Geometry: final body of the model. Coordinates: model frame, mm. Face numbers are marked on the shaded views. A direction names the side the tool comes from. Coordinates: 2 decimals unless noted, no trailing zeros. Write each loop counter-clockwise with the first axis right and the second up, starting at its lowest first coordinate (ties: lowest second). Pieces come first, ordered by that corner, then holes.
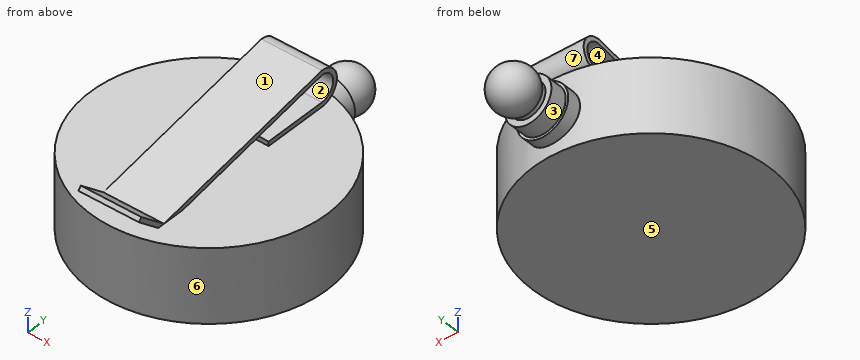
from build123d import *

# Parameters (mm, degrees)
F0_R     = 16
F1_DEPTH = 10
F3_DEPTH = 4.1


with BuildPart() as f1:
    # F0 (on Top) → F1 (new body)
    with BuildSketch(Plane.XY):
        Circle(F0_R)
    extrude(amount=F1_DEPTH)

    # F2 (on Right) → F3 (join, symmetric)
    with BuildSketch(Plane.YZ):
        with BuildLine():
            Line((4.757335, 10.697019), (4.757335, 10.097019))
            Line((4.757335, 10.097019), (13.346032, 10.097019))
            ThreePointArc((13.346032, 10.097019), (15.746032, 12.497019), (13.346032, 14.897019))
            Line((13.346032, 14.897019), (-12.123428, 10.016164))
            Line((-12.123428, 10.016164), (-15.761921, 13.08867))
            Line((-15.761921, 13.08867), (-16.14903, 12.630252))
            Line((-16.14903, 12.630252), (-12.291747, 9.37299))
            Line((-12.291747, 9.37299), (13.398945, 14.296242))
            ThreePointArc((13.398945, 14.296242), (15.145838, 12.47056), (13.346032, 10.697019))
            Line((13.346032, 10.697019), (4.757335, 10.697019))
        make_face()
    extrude(amount=F3_DEPTH, both=True)

    # F5 (on offset) → F6 (revolve)
    with BuildSketch(Plane.XY.offset(5)):
        with BuildLine():
            Line((-3.5, 15.612495), (0, 15.612495))
            Line((0, 15.612495), (0, 25.177301))
            ThreePointArc((0, 25.177301), (-2.701335, 23.482211), (-2.35, 20.312495))
            Line((-2.35, 20.312495), (-2.35, 19.812495))
            Line((-2.35, 19.812495), (-3.15, 19.812495))
            Line((-3.15, 19.812495), (-3.15, 17.512495))
            Line((-3.15, 17.512495), (-3.5, 17.512495))
            Line((-3.5, 17.512495), (-3.5, 15.612495))
        make_face()
    revolve(axis=Axis((0, 20.394898, 5), (0, -1, 0)))


solid = f1.part
Item 1: Set-up query: the marked faces 1, 2 and 3. Return all of +Z, -Z, +X, -X, +Y, -Y with unobstructed straight access to the full face (end or side cutting, diameter ignored); none if empty.
Derived:
face 1: +Z, +X, -X
face 2: +X, -X
face 3: +Y
Item 2: Pull-direction query (Y, two-part tool) for the marked faces 4, 5, 6 and 7; classes: released by +Y, released by -Y, zero draft, split by the parting line, or undercut.
Derived:
face 4: undercut
face 5: zero draft
face 6: split by the parting line
face 7: released by +Y
Item 3: Section A-A, the plane y = -5. Output: boundary loops of the cut face in (x, z), plus the area to 3 significant figures.
Derived:
outline: (-15.2, 0) - (15.2, 0) - (15.2, 10) - (-15.2, 10) - close; (-4.1, 10.77) - (4.1, 10.77) - (4.1, 11.38) - (-4.1, 11.38) - close
area: 309 mm2
Item 4: Section D-D, the plane y = 0. Output: boundary loops of the cut face in (x, z), plus the area to 3 significant figures.
Derived:
outline: (-16, 0) - (16, 0) - (16, 10) - (-16, 10) - close; (-4.1, 11.73) - (4.1, 11.73) - (4.1, 12.34) - (-4.1, 12.34) - close
area: 325 mm2
Item 5: Pin query (flat end, axial travel): pin 1 (5 mm diameter, centred on x = 3.5, y = -4, fed in from +Z); pin 2 (1 mm diameter, centred on x = -7.5, z = 3.5, fed in from +Y); pin 3 (6 mm diameter, centred on y = 14, z = 6, fed in from -X). Return the tip coordinate at first contact, or that it passes through.
Derived:
pin 1: stops at z = 12.05
pin 2: stops at y = 14.39
pin 3: stops at x = -11.62
Item 6: Material intervals for probe 1 along Z at (x, y) = (-8, -7); probe 2 along Y at (x, z) = (-10, 1); probe 3 along X at (y, z) = (4, 4), sorted ascending.
Derived:
probe 1: z = 0 to 10
probe 2: y = -12.49 to 12.49
probe 3: x = -15.49 to 15.49
Item 7: Section C-C, the plane x = -7.5. Output: boundary loops of the cut face in (y, z), plus the area to 3 significant figures.
Derived:
outline: (-14.13, 0) - (14.13, 0) - (14.13, 10) - (-14.13, 10) - close
area: 283 mm2
Item 8: Section B-B, the plane y = 7. Output: boundary loops of the cut face in (x, z), plus the area to 3 significant figures.
Derived:
outline: (-14.39, 0) - (14.39, 0) - (14.39, 10) - (-14.39, 10) - close; (-4.1, 10.1) - (4.1, 10.1) - (4.1, 10.7) - (-4.1, 10.7) - close; (-4.1, 13.07) - (4.1, 13.07) - (4.1, 13.68) - (-4.1, 13.68) - close
area: 298 mm2
